Model file for the job. Use its own axes, mm. A direction names the side the tool comes from. Round coordinates to 2 decimals unless told otherwise and drop trailing zeros. Write each loop counter-clockwise with the first axis right and the second up, starting at its lowest first coordinate (ties: lowest second). Pieces come first, ordered by that corner, then holes.
```python
from build123d import *

# Parameters (mm, degrees)
ESQUISSE1_W             = 40.3
ESQUISSE1_H             = 20.2
BOSS_EXTRU_1_DEPTH      = 32.1
ESQUISSE2_W             = 54
ESQUISSE2_H             = 20.2
BOSS_EXTRU_2_DEPTH      = 2
ESQUISSE3_W             = 40.3
ESQUISSE3_H             = 20.2
BOSS_EXTRU_3_DEPTH      = 10.8
ESQUISSE4_R             = 3
BOSS_EXTRU_4_DEPTH      = 4
ESQUISSE5_R             = 2.5
ENL_V_MAT_EXTRU_1_DEPTH = 4


with BuildPart() as part:
    # Esquisse1 → Boss.-Extru.1 (new body)
    with BuildSketch(Plane.XY):
        with Locations((20.15, 5.491176471)):
            Rectangle(ESQUISSE1_W, ESQUISSE1_H)
    extrude(amount=BOSS_EXTRU_1_DEPTH)

    # Esquisse2 → Boss.-Extru.2 (add)
    with BuildSketch(Plane.XY.offset(32.1)):
        with Locations((20.15, 5.491176471)):
            Rectangle(ESQUISSE2_W, ESQUISSE2_H)
    extrude(amount=BOSS_EXTRU_2_DEPTH)

    # Esquisse3 → Boss.-Extru.3 (add)
    with BuildSketch(Plane.XY.offset(34.1)):
        with Locations((20.15, 5.491176471)):
            Rectangle(ESQUISSE3_W, ESQUISSE3_H)
    extrude(amount=BOSS_EXTRU_3_DEPTH)

    # Esquisse4 → Boss.-Extru.4 (add)
    with BuildSketch(Plane.XY.offset(44.9)):
        with Locations(Location((9.85, 5.491176471, 0), (0, 0, 180))):
            Circle(ESQUISSE4_R)
    extrude(amount=BOSS_EXTRU_4_DEPTH)

    # Esquisse5 → Enlèv. mat.-Extru.1 (cut)
    with BuildSketch(Plane.XY.offset(34.1)):
        with Locations((-3.88, 10.591176471)):
            Circle(ESQUISSE5_R)
        with Locations((-3.832055369, 0.591291406)):
            Circle(ESQUISSE5_R)
        with Locations((44.12, 10.591176471)):
            Circle(ESQUISSE5_R)
        with Locations((44.167944631, 0.591291406)):
            Circle(ESQUISSE5_R)
    extrude(amount=-ENL_V_MAT_EXTRU_1_DEPTH, mode=Mode.SUBTRACT)


solid = part.part
```
1) Cut at A-A on y = 9.75. List the corners of the cut face in (x, z).
2) Wall check: probe 1 along Y at (x, z) = (44, 33); probe 2 along Z at (x, y) = (23, 12.25); probe 3 along X at (y, z) = (14.5, 37). Give the ranges that are in metal, low to high.
3) Cut at D-D on z = 29.5. List the corners of the cut face in (x, y).
4) Which spindle directions (+Z, -Z, +X, -X, +Y, -Y) get a long thin tool onto all of the face, cutting with end or side? Do faces 5 (the face through (0, 5, 16)), 6 (the face through (40.3, 5, 39)), 7 (the face through (44, 6, 32.1)). Say none if no direction does.
5) Flat gauge pins, fed straight in: pin 1 Ø7.5 at (x, y) = (-3, 6) entering from +Z; pin 2 Ø6 at (y, z) = (8, 20) entering from -X; pin 3 Ø1.5 at (x, y) = (40, 8.5) entering from -Z; pin 4 Ø2 at (x, y) = (-2, 6.5) entering from -Z. Where does each tip first touch, or does it go through?
6) Pull direction Y, two halves, no side cores. Call faces 1 (the face through (20, 15.591, 22)), 2 (the face through (41.622, 10.701, 33.114)), 3 (the face through (47.15, 5, 33)), 4 (the face through (10.241, 2.517, 46.872)): released by +Y, released by -Y, zero draft, split by the parting line, or undercut.
7) Cut at B-B on x = 9.85. List the corners of the cut face in (y, z), and give its area (3 significant figures).
8) Cut at C-C on x = 44.12. List the corners of the cut face in (y, z).
Result sheet:
1. outline: (-6.85, 32.1) - (-6.23, 32.1) - (-6.23, 34.1) - (-6.85, 34.1) - close; (-1.53, 32.1) - (0, 32.1) - (0, 0) - (40.3, 0) - (40.3, 32.1) - (41.77, 32.1) - (41.77, 34.1) - (40.3, 34.1) - (40.3, 44.9) - (0, 44.9) - (0, 34.1) - (-1.53, 34.1) - close; (46.47, 32.1) - (47.15, 32.1) - (47.15, 34.1) - (46.47, 34.1) - close
2. probe 1: y = -4.61 to -1.9, 3.09 to 8.09, 13.09 to 15.59
2. probe 2: z = 0 to 44.9
2. probe 3: x = 0 to 40.3
3. outline: (0, -4.61) - (40.3, -4.61) - (40.3, 15.59) - (0, 15.59) - close
4. face 5: -Z, -X, +Y, -Y
4. face 6: +Z, +X, +Y, -Y
4. face 7: -Z, +X, +Y, -Y
5. pin 1: stops at z = 44.9
5. pin 2: stops at x = 0
5. pin 3: stops at z = 0
5. pin 4: stops at z = 32.1
6. face 1: released by +Y
6. face 2: undercut
6. face 3: zero draft
6. face 4: split by the parting line
7. outline: (-4.61, 0) - (15.59, 0) - (15.59, 44.9) - (8.49, 44.9) - (8.49, 48.9) - (2.49, 48.9) - (2.49, 44.9) - (-4.61, 44.9) - close
7. area: 931 mm2
8. outline: (-4.61, 32.1) - (-1.91, 32.1) - (-1.91, 34.1) - (-4.61, 34.1) - close; (3.09, 32.1) - (8.09, 32.1) - (8.09, 34.1) - (3.09, 34.1) - close; (13.09, 32.1) - (15.59, 32.1) - (15.59, 34.1) - (13.09, 34.1) - close
